Autodesk Inventor part; units mm, degrees
ref_plane "Work Plane1" through (0, 2.921, -2.54) normal (0, 1, 0) x (-1, 0, 0)
ref_plane "YZ Plane" through (0, 0, 0) normal (1, 0, 0) x (0, 1, 0)
ref_plane "XZ Plane" through (0, 0, 0) normal (0, 1, 0) x (-1, 0, 0)
sketch "Sketch1" plane through (0, 0, 0) normal (0, 0, 1) x (1, 0, 0)
  circle A0 centre (0, 0) radius 2.921
  dimension "d0" = 5.842
extrude "Extrusion1" add sketch "Sketch1" along normal blind 12.7
sketch "Sketch2" plane through (0, 0, 12.7) normal (0, 0, 1) x (1, 0, 0)
  circle A0 centre (0, 0) radius 3.81
  dimension "d3" = 7.62
extrude "Extrusion2" add sketch "Sketch2" along normal blind 2.54
sketch "Sketch3" plane through (0, 0, 0) normal (0, 0, -1) x (-1, 0, 0)
  circle A0 centre (0, 0) radius 2.921
  dimension "d12" = 5.842
extrude "Extrusion3" add sketch "Sketch3" along normal blind 2.54
sketch "Sketch4" plane through (0, 0, -2.54) normal (0, 0, -1) x (-1, 0, 0)
  circle A0 centre (0, 0) radius 2.921
  point P0 (0, 2.921)
ref_plane "Work Plane1" through (0, 2.921, -2.54) normal (0, 1, 0) x (-1, 0, 0)
sketch "Sketch5" plane through (0, 2.921, -2.54) normal (0, 1, 0) x (-1, 0, 0)
  circle A0 centre (0, 1.27) radius 0.885
  line L0 (-2.921, 0) -> (2.921, 0)
  point P0 (0, 2.54)
  dimension "d8" = 1.77
  dimension "d9" = 1.27
extrude "Extrusion4" cut sketch "Sketch5" against normal blind 7.3025
properties part number "Pin"
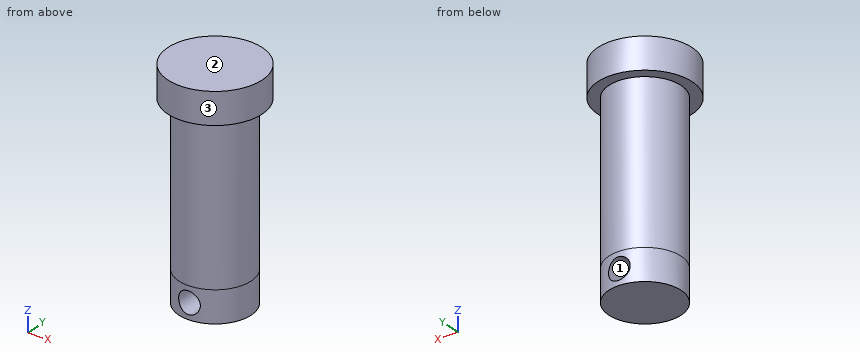
Source: CAD feature listing. Evaluate the final solid. Frame: model axes, mm. Face numbers are marked on the shaded views. Round coordinates to 2 decimals unless told otherwise and drop trailing zeros. Loops run counter-clockwise (first coordinate to the right, second up) from the corner with the lowest first, then second, coordinate; pieces in that order, holes last. Notation, with made-up numbers: M 41.5,2.25 L 86.5,2.25 A8 ccw 86.5,11.25 Z; hole C -15.75,34 d5. An arc over 180 degrees is marked long. Put each result on its own line as item: value.
(1) First-contact query: pin 1 (2 mm diameter, centred on y = 1.5, z = 4.5, fed in from -X); pin 2 (4 mm diameter, centred on y = 3, z = 4, fed in from +X); pin 3 (4 mm diameter, centred on y = 3, z = 1, fed in from -X). Flat tips, straight axial feed; report the tip coordinate or a pass-through.
Solutions:
pin 1: x = -2.88
pin 2: x = 2.74
pin 3: x = -2.74
(2) Pull-direction query (X, two-part tool) for the marked faces 1, 2 and 3; classes: released by +X, released by -X, zero draft, split by the parting line, or undercut.
Solutions:
face 1: undercut
face 2: zero draft
face 3: split by the parting line
(3) Section D-D, the plane z = 11.5. Return loops of the section in (x, y), and give its area (3 significant figures).
Solutions:
outline: C 0,0 d5.84
area: 26.8 mm²
(4) Section A-A, the plane x = 0. Return loops of the section in (y, z) (3 decimals), and give its area (3 significant figures).
Solutions:
outline: M -3.81,12.7 L -2.921,12.7 L -2.921,-0.385 L 2.921,-0.385 L 2.921,12.7 L 3.81,12.7 L 3.81,15.24 L -3.81,15.24 Z; M -2.921,-2.54 L 2.921,-2.54 L 2.921,-2.155 L -2.921,-2.155 Z
area: 98.0 mm²
(5) Ray query, line 1 (Z direction, x = 0, y = -0.85) (3 decimals); line 2 (X direction, y = 0.1, z = -1.27) (3 decimals); line 3 (Z direction, x = -3.5, y = 1). Return the intervals inside material, ascending. Write a range as [from, to].
Solutions:
line 1: [-2.54, -2.155], [-0.385, 15.24]
line 2: [-2.919, -0.885], [0.885, 2.919]
line 3: [12.7, 15.24]
(6) Section C-C, the plane y = -2.25. Return loops of the section in (x, z) (3 decimals), and give its area (3 significant figures).
Solutions:
outline: M -3.075,12.7 L -1.863,12.7 L -1.863,-2.54 L 1.863,-2.54 L 1.863,12.7 L 3.075,12.7 L 3.075,15.24 L -3.075,15.24 Z; hole C 0,-1.27 d1.77
area: 69.9 mm²
(7) Section B-B, the plane y = 0. Return loops of the section in (x, z) (3 decimals).
Solutions:
outline: M -3.81,12.7 L -2.921,12.7 L -2.921,-2.54 L 2.921,-2.54 L 2.921,12.7 L 3.81,12.7 L 3.81,15.24 L -3.81,15.24 Z; hole C 0,-1.27 d1.77
